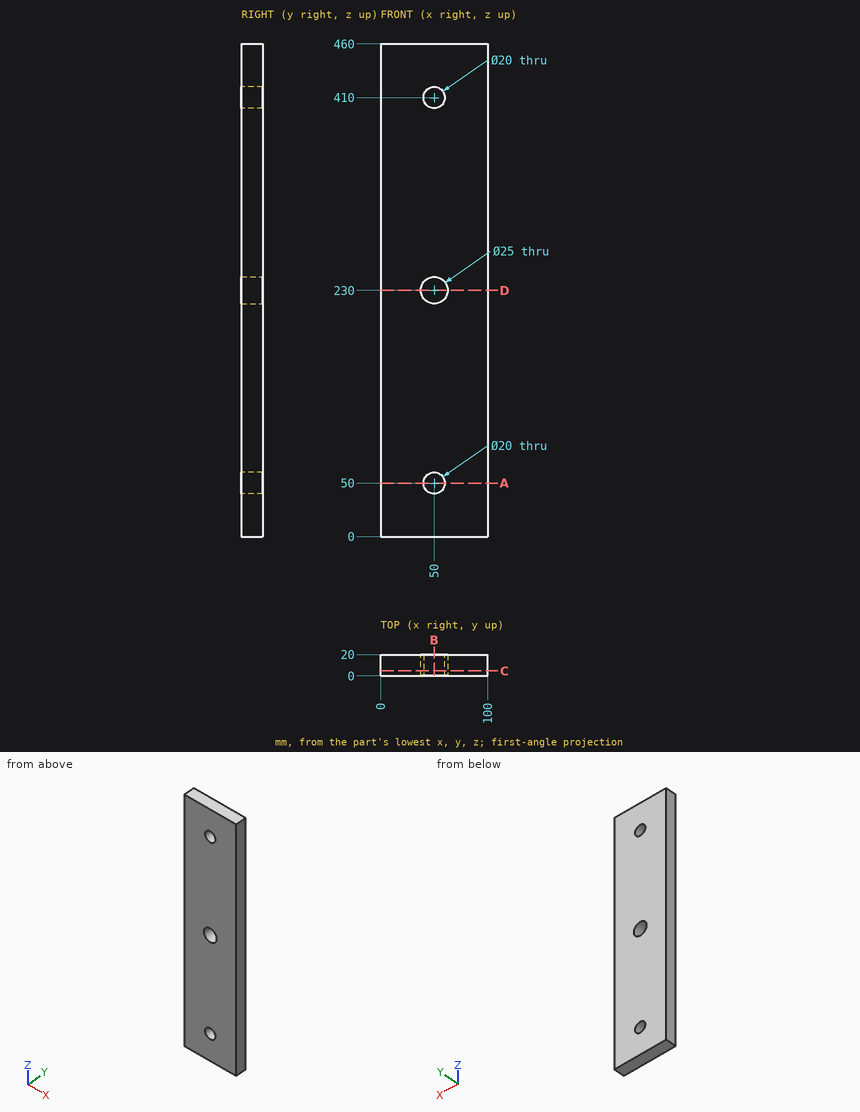
For this review, use the dimensioned drawing (mm, ordinates from the lowest corner) and the shaded views. Give positions to 0.01 mm unless a question says otherwise; leave off trailing zeros. Order: outer loops, then holes, each group sorted by start corner. A loop starts at its lowest first (then second) coordinate and runs counter-clockwise, first axis right, second up. Notation, with made-up numbers: (-37, 23.25) - (-31, 23.25) arc R21 cw to (-31, 41.25) - close; hole circle Ø1 at (45, 64.5). An arc over 180 degrees is marked (long way). Write item = value, one per line. Start each with the question number.
Q1. We need section D-D on z = 230. State the section outline as (x, y) points.
Q2. We need section B-B on x = 50. State the section outline as (y, z) points, plus the area to 3 significant figures.
Q3. We need section A-A on z = 50. State the section outline as (x, y) points, plus the area to 3 significant figures.
Q4. To check wall thickness, follow L1, parallel to Z at x = 50, y = 8; L2, parallel to X at y = 4.5, z = 50; L3, parallel to Z at x = 45, y = 8.25. State the ranges of each line that lie inside material, in increasing order. Write a range as from..to.
Q5. We need section C-C on y = 4.75. State the section outline as (x, z) points.
Working result:
q1.outline = (0, 0) - (37.5, 0) - (37.5, 20) - (0, 20) - close; (62.5, 0) - (100, 0) - (100, 20) - (62.5, 20) - close
q2.outline = (0, 0) - (20, 0) - (20, 40) - (0, 40) - close; (0, 60) - (20, 60) - (20, 217.5) - (0, 217.5) - close; (0, 242.5) - (20, 242.5) - (20, 400) - (0, 400) - close; (0, 420) - (20, 420) - (20, 460) - (0, 460) - close
q2.area = 7,900 mm²
q3.outline = (0, 0) - (40, 0) - (40, 20) - (0, 20) - close; (60, 0) - (100, 0) - (100, 20) - (60, 20) - close
q3.area = 1,600 mm²
q4.L1 = 0..40, 60..217.5, 242.5..400, 420..460
q4.L2 = 0..40, 60..100
q4.L3 = 0..41.34, 58.66..218.54, 241.46..401.34, 418.66..460
q5.outline = (0, 0) - (100, 0) - (100, 460) - (0, 460) - close; hole circle Ø25 at (50, 230); hole circle Ø20 at (50, 50); hole circle Ø20 at (50, 410)
